Design review of the part built by this model. Coordinates are the model's own, in mm. Face numbers are marked on the shaded views. A direction names the side the tool comes from. Coordinates: 2 decimals unless noted, no trailing zeros. Write each loop counter-clockwise with the first axis right and the second up, starting at its lowest first coordinate (ties: lowest second). Pieces come first, ordered by that corner, then holes. Notation, with made-up numbers: (25, 14) - (50, 14) arc R19 cw to (50, 42) - close; hole circle Ø5 at (55.5, 52.25). An arc over 180 degrees is marked (long way). Answer as CSV lines item,"result". Start each with the question number.
Q1. We need section C-C (y = -0.5). Write out the cut boundary in (x, z).
Q2. We need section D-D (x = 15). Write out the cut boundary in (y, z).
Q3. Mouldability with a two-part tool opening along Y and no side actions: class the marked faces 3, 4 and 5 as pulls with the +Y half, pulls with the -Y half, needs draft (parallel to the pull), parting line crosses it, or undercut.
Q4. We need section B-B (z = 0.55). Write out the cut boundary in (x, y).
Q5. We need section A-A (x = 13). Write out the cut boundary in (y, z), plus the area to 3 significant figures.
Q6. Machinability: for the marked faces 1 and 2, which of the approach directions +Z, -Z, +X, -X, +Y, -Y give a long, thin tool a straight path to every point of the face, cutting with its end or side? Answer none if there is none.
Q7. Clearance check with a flat-ended pin moving along its axis: pin 1 (1 mm diameter, centred on x = 13, y = -5.5, fed in from -Z). State where the tip first meets the part, or that it passes through.
Q8. For line 1 along Y through (x, z) = (9.25, 1.1); line 2 along Y through (x, z) = (14.75, 0.95); line 3 along X through (y, z) = (-4.25, 0.95), list the stretches that pass through material, from the lowest coordinate up. Write a range as [from, to].
from build123d import *

# Parameters (mm, degrees)
SM_BASE_FLANGE_1_DEPTH = 1.4
FILLET_1_R             = 0.2


# Sheet-metal steps are written as plain solids
with BuildPart() as part:
    # Sketch 1 → Базовая кромка1 (new body)
    with BuildSketch(Plane.XY):
        with BuildLine():
            Line((0, 0), (14, 0))
            ThreePointArc((14, 0), (16.121320344, -0.878679656), (17, -3))
            Line((17, -3), (17, -3.5))
            ThreePointArc((17, -3.5), (16.121320344, -5.621320344), (14, -6.5))
            Line((14, -6.5), (0, -6.5))
            Line((0, -6.5), (0, -5.8))
            Line((0, -5.8), (14, -5.8))
            ThreePointArc((14, -5.8), (15.626345597, -5.126345597), (16.3, -3.5))
            Line((16.3, -3.5), (16.3, -3))
            ThreePointArc((16.3, -3), (15.626345597, -1.373654403), (14, -0.7))
            Line((14, -0.7), (0, -0.7))
            Line((0, -0.7), (0, 0))
        make_face()
    extrude(amount=SM_BASE_FLANGE_1_DEPTH)

    # Скругление1
    fillet_1_edges = [part.edges().sort_by_distance(p)[0] for p in [
        (0, -0.35, 0),
        (0, -6.15, 0),
        (0, -0.35, 1.4),
        (0, -6.15, 1.4),
    ]]
    fillet(fillet_1_edges, radius=FILLET_1_R)


solid = part.part
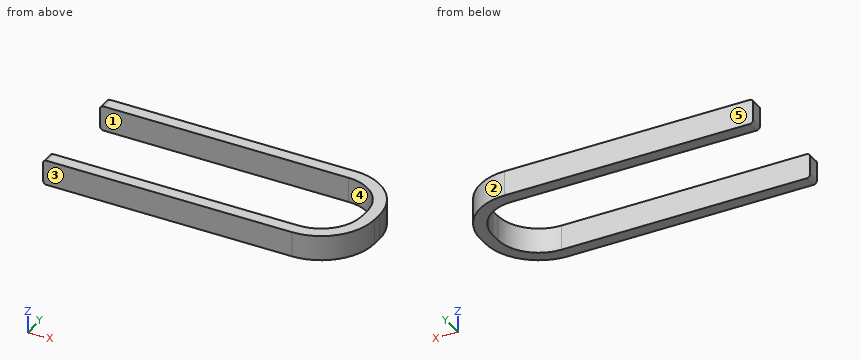
Results list:
1,outline,"(0, 0.2) arc R0.2 ccw to (0.2, 0) - (15.66, 0) - (15.66, 1.4) - (0.2, 1.4) arc R0.2 ccw to (0, 1.2) - close"
2,outline,"(-6.33, 0) - (-5.57, 0) - (-5.57, 1.4) - (-6.33, 1.4) - close; (-0.93, 0) - (-0.17, 0) - (-0.17, 1.4) - (-0.93, 1.4) - close"
3,face 3,"pulls with the -Y half"
3,face 4,"undercut"
3,face 5,"pulls with the +Y half"
4,outline,"(0, -6.5) - (14, -6.5) arc R3 ccw to (17, -3.5) - (17, -3) arc R3 ccw to (14, 0) - (0, 0) - (0, -0.7) - (14, -0.7) arc R2.3 cw to (16.3, -3) - (16.3, -3.5) arc R2.3 cw to (14, -5.8) - (0, -5.8) - close"
5,outline,"(-6.5, 0) - (-5.8, 0) - (-5.8, 1.4) - (-6.5, 1.4) - close; (-0.7, 0) - (0, 0) - (0, 1.4) - (-0.7, 1.4) - close"
5,area,"1.96 mm2"
6,face 1,"+Z, -Z, -X"
6,face 2,"+Z, -Z, +X, +Y"
7,pin 1,"stops at z = 0"
8,line 1,"y = [-6.5, -5.8], [-0.7, 0]"
8,line 2,"y = [-6.4, -5.67], [-0.83, -0.1]"
8,line 3,"x = [16.17, 16.9]"
